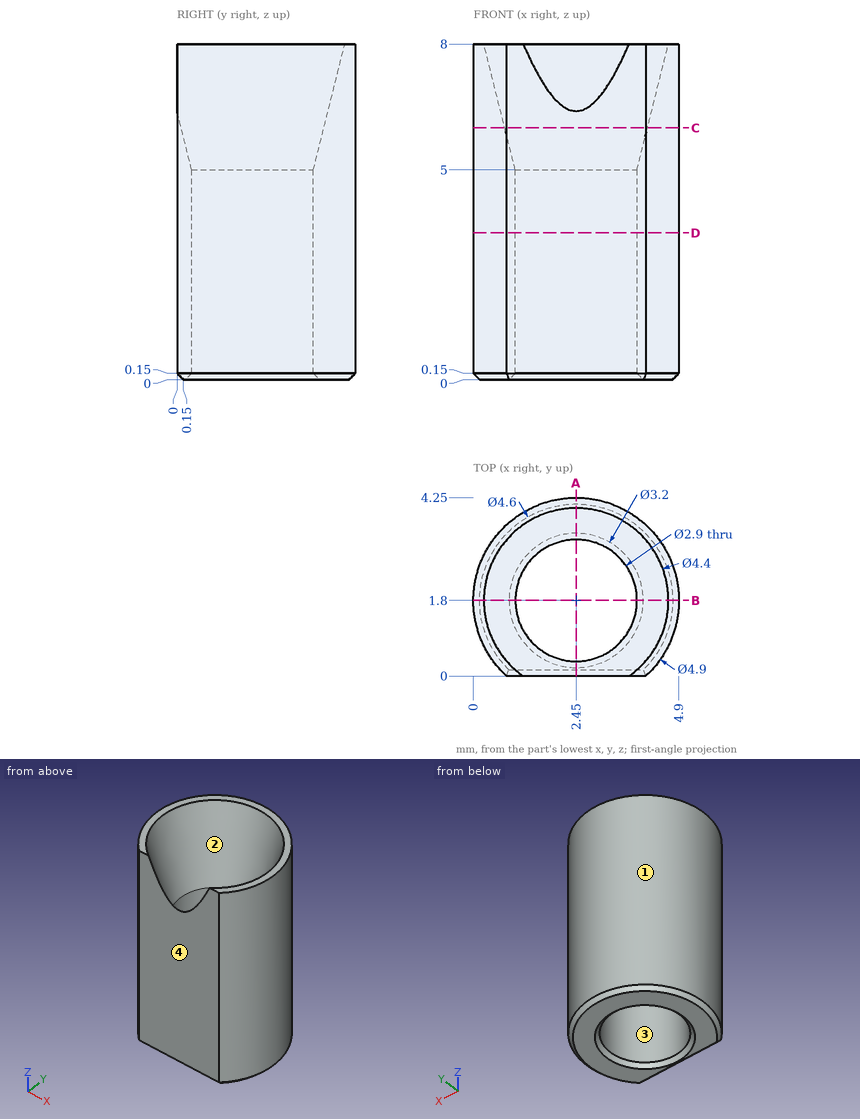
Answer from the drawing. Dimensions are ordinates in mm from the lowest x, y and z of the part. Give positions to 0.01 mm unless a question says otherwise; leave off trailing zeros. Order: outer loops, then holes, each group sorted by start corner. A loop starts at its lowest first (then second) coordinate and runs counter-clockwise, first axis right, second up.
Item 1: Given pin 1 Ø2 at (x, z) = (1, 4.5) entering from +Y, flat-ended and moving along its own axis, determine where the tip first touches the part or whether it passes through.
From the geometry:
pin 1: stops at y = 4.21
Item 2: Find the intervals of material crossed by probe 1 along Y at (x, z) = (1.8, 4.5); probe 2 along X at (y, z) = (2.1, 3.5); probe 3 along X at (y, z) = (1.1, 4.5), in increasing order.
From the geometry:
probe 1: y = 0 to 0.5, 3.1 to 4.16
probe 2: x = 0.02 to 1.03, 3.87 to 4.88
probe 3: x = 0.1 to 1.18, 3.72 to 4.8
Item 3: For a pull along Y with two mould halves and no side action, classify the marked faces 1, 2, 3 and 4 as pulls with the +Y half, pulls with the -Y half, needs draft (parallel to the pull), parting line crosses it, or undercut.
From the geometry:
face 1: parting line crosses it
face 2: undercut
face 3: undercut
face 4: pulls with the -Y half
Item 4: The part is cut by section C-C, the plane z = 6. Give the vertices of the cut face in (x, y).
From the geometry:
outline: (0.79, 0) - (4.11, 0) arc R2.45 ccw (long way) to start; hole circle Ø3.4 at (2.45, 1.8)
Item 5: The part is cut by section D-D, the plane z = 3.5. Give the vertices of the cut face in (x, y).
From the geometry:
outline: (0.79, 0) - (4.11, 0) arc R2.45 ccw (long way) to start; hole circle Ø2.9 at (2.45, 1.8)
Item 6: The part is cut by section B-B, the plane y = 1.8. Give the vertices of the cut face in (x, z).
From the geometry:
outline: (0, 0.15) - (0.15, 0) - (0.85, 0) - (1, 0.15) - (1, 5) - (0.25, 8) - (0, 8) - close; (3.9, 0.15) - (4.05, 0) - (4.75, 0) - (4.9, 0.15) - (4.9, 8) - (4.65, 8) - (3.9, 5) - close
Item 7: The part is cut by section A-A, the plane x = 2.45. Give the vertices of the cut face in (y, z), and give its area (4 significant figures).
From the geometry:
outline: (0, 0.15) - (0.15, 0) - (0.2, 0) - (0.35, 0.15) - (0.35, 5) - (0, 6.4) - close; (3.25, 0.15) - (3.4, 0) - (4.1, 0) - (4.25, 0.15) - (4.25, 8) - (4, 8) - (3.25, 5) - close
area: 8.825 mm2
